from build123d import *

# Parameters (mm, degrees)
SKETCH_R      = 6
SKETCH_R_2    = 5.25
PAD_DEPTH     = 25
SKETCH001_R   = 7
SKETCH001_R_2 = 5.25
PAD001_DEPTH  = 2
FILLET_R      = 1


with BuildPart() as part:
    # Sketch → Pad (new body)
    with BuildSketch(Plane.XY):
        Circle(SKETCH_R)
        Circle(SKETCH_R_2, mode=Mode.SUBTRACT)
    extrude(amount=PAD_DEPTH)

    # Sketch001 (on Face4 of Pad) → Pad001 (join)
    with BuildSketch(Plane.XY.offset(25)):
        Circle(SKETCH001_R)
        Circle(SKETCH001_R_2, mode=Mode.SUBTRACT)
    extrude(amount=PAD001_DEPTH)

    # Fillet
    fillet_edges = [part.edges().sort_by_distance(p)[0] for p in [
        (-5.25, 0, 27),
    ]]
    fillet(fillet_edges, radius=FILLET_R)


solid = part.part
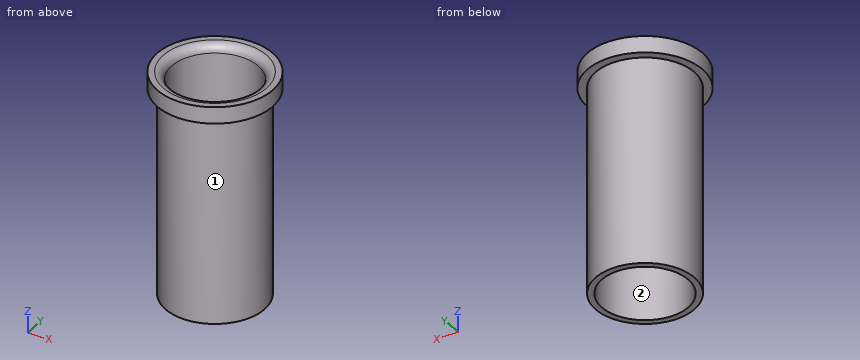
Geometry: final body of the model. Coordinates: model frame, mm. Face numbers are marked on the shaded views. Give positions to 0.01 mm unless a question says otherwise; leave off trailing zeros. Write each loop counter-clockwise with the first axis right and the second up, starting at its lowest first coordinate (ties: lowest second). Pieces come first, ordered by that corner, then holes. Notation, with made-up numbers: (12, 59.5) - (53, 59.5) arc R21 ccw to (53, 75.5) - close; hole circle Ø6 at (44, -17.5). An arc over 180 degrees is marked (long way). Return JSON: item names as keys, results as strings. Group by question number.
1) Line query: line 1 (Y direction, x = 0, z = 6); line 2 (Z direction, x = 5.25, y = -4); line 3 (X direction, y = 4, z = 11.75). Output: solid intervals per line, ascending.
2) Mould query, pull axis X, two halves, no side actions, for the marked faces 1 and 2. Classes: released by +X, released by -X, zero draft, split by the parting line, or undercut.
3) Section C-C on z = 5. Return the cut outline in (x, y), plus the area to 3 significant figures.
4) Section A-A on y = 0. Return the cut outline in (x, z), plus the area to 3 significant figures.
5) First-contact query: P1, Ø1.5, axis at y = -2, z = 6, coming from the +X side; P2, Ø1, axis at y = 2.5, z = 18, coming from the +X side; P3, Ø8, axis at x = -2, y = 4.5, coming from the +Z side; P4, Ø5, axis at x = -5, z = 20, coming from the +Y side. Flat tips, straight axial feed; report the tip coordinate or a pass-through.
Filled in:
{
 "1": {"line 1": "y = -6 to -5.25, 5.25 to 6", "line 2": "z = 25 to 27", "line 3": "x = -4.47 to -3.4, 3.4 to 4.47"},
 "2": {"face 1": "split by the parting line", "face 2": "undercut"},
 "3": {"outline": "circle Ø12 at (0, 0); hole circle Ø10.5 at (0, 0)", "area": "26.5 mm^2"},
 "4": {"outline": "(-7, 25) - (-6, 25) - (-6, 0) - (-5.25, 0) - (-5.25, 26) arc R1 ccw to (-6.25, 27) - (-7, 27) - close; (5.25, 0) - (6, 0) - (6, 25) - (7, 25) - (7, 27) - (6.25, 27) arc R1 ccw to (5.25, 26) - close", "area": "44.1 mm^2"},
 "5": {"P1": "stops at x = 5.87", "P2": "stops at x = 5.66", "P3": "stops at z = 27", "P4": "stops at y = 5.45"}
}
